Read the model definition and answer for the solid it produces. Units are mm, in the model's axes. A direction names the side the tool comes from. Coordinates: 2 decimals unless noted, no trailing zeros. Write each loop counter-clockwise with the first axis right and the second up, starting at its lowest first coordinate (ties: lowest second). Pieces come first, ordered by that corner, then holes.
1) Determine the mould class of faces 1 (the face through (131.79, 7.81, -1.73)), 2 (the face through (0, 17, -17)), 3 (the face through (96, 0, -11)) for opening direction X: +X half, -X half, draft (parallel to the pull), parting line (faces both ways), or undercut.
2) Each of these flat-tipped pins is pushed along its axis until it touches: pin 1 Ø10 at (x, z) = (55.5, 20.5) entering from -Y; pin 2 Ø16 at (x, y) = (91, -7) entering from +Z; pin 3 Ø4 at (x, z) = (100, 21) entering from +Y. Where does it stop, or does it pass through?
3) Which of the six approach directions +Z, -Z, +X, -X, +Y, -Y give full straight-line access (tool end or side, diameter ignored) to faces 4 (the face through (110, 16, 12)), 5 (the face through (110, -16, 12)), 6 (the face through (89.649, 0.528, 23.994))?
4) The part is cut by section A-A (x = 111.5). Determine the outline of the cut face in (y, z), then the cut area to 3 significant figures.
5) Find the intervals of material crossed by line 1 (Y direction, x = 133.25, z = 0); line 2 (Z direction, x = 45, y = 16); line 3 (Y direction, x = 56.75, z = 0), in increasing order.
6) The part is cut by section D-D (x = 26). Determine the outline of the cut face in (y, z).
7) The part is cut by section C-C (z = -5.5). Give the number of separate pieces and of enclosed holes in the cut face, then the cut area to 3 significant figures.
8) The part is cut by section B-B (y = 0). Determine the outline of the cut face in (x, z).
from build123d import *

# Parameters (mm, degrees)
CUT_EXTRUDE1_DEPTH = 151.996688705
SKETCH4_W          = 57
SKETCH4_H          = 22
CUT_EXTRUDE2_DEPTH = 156.357021604


with BuildPart() as part:
    # Sketch1 → Revolve1 (revolve)
    with BuildSketch(Plane(origin=(0, 0, 0), x_dir=(1, 0, 0), z_dir=(0, 1, 0)), mode=Mode.PRIVATE) as revolve1_sk:
        with BuildLine():
            Line((0, 0), (0, 40))
            Line((0, 40), (45, 24))
            Line((45, 24), (133.065732621, 24))
            ThreePointArc((133.065732621, 24), (138.23168958, 12.490837283), (140, 0))
            Line((140, 0), (0, 0))
        make_face()
    revolve(revolve1_sk.sketch.rotate(Axis((0, 0, 0), (1, 0, 0)), 180), axis=Axis((0, 0, 0), (1, 0, 0)))

    # Sketch2 → Cut-Extrude1 (cut, symmetric)
    with BuildSketch(Plane.XY):
        Polygon((469.549791622, 16), (137.05948169, 16), (67.5, 16), (0, 40), (-313.277254393, 151.387468229), (-199.953261752, 806.640776108), (582.873784263, 671.253307879), align=None)
    cut_extrude1 = extrude(amount=CUT_EXTRUDE1_DEPTH, both=True, mode=Mode.SUBTRACT)

    # Mirror1: Cut-Extrude1 across plane
    add(cut_extrude1.mirror(Plane.ZX), mode=Mode.SUBTRACT)

    # Sketch3 → Cut-Revolve2 (revolve, cut)
    with BuildSketch(Plane(origin=(0, 0, 0), x_dir=(1, 0, 0), z_dir=(0, 1, 0)), mode=Mode.PRIVATE) as cut_revolve2_sk:
        Polygon((0, 23.01873218), (0, 0), (140, 0), (140, 8), (42.240184255, 8), align=None)
    revolve(cut_revolve2_sk.sketch.rotate(Axis((0, 0, 0), (1, 0, 0)), 180), axis=Axis((0, 0, 0), (1, 0, 0)), mode=Mode.SUBTRACT)

    # Sketch4 → Cut-Extrude2 (cut, through all)
    with BuildSketch(Plane(origin=(0, 16, 0), x_dir=(1, 0, 0), z_dir=(0, 1, 0))):
        with Locations((96, 0)):
            Rectangle(SKETCH4_W, SKETCH4_H)
    extrude(amount=-CUT_EXTRUDE2_DEPTH, mode=Mode.SUBTRACT)


solid = part.part
Reported:
1. face 1: draft
1. face 2: -X half
1. face 3: undercut
2. pin 1: stops at y = -18.32
2. pin 2: stops at z = 24
2. pin 3: stops at y = 14.66
3. face 4: +Z, -Z, +X, +Y
3. face 5: +Z, -Z, +X, -Y
3. face 6: +Z, +X
4. outline: (-16, -17.89) arc R24 ccw to (16, -17.89) - (16, -11) - (-16, -11) - close; (-16, 11) - (16, 11) - (16, 17.89) arc R24 ccw to (-16, 17.89) - close
4. area: 709 mm2
5. line 1: y = -16 to -8, 8 to 16
5. line 2: z = -17.89 to 17.89
5. line 3: y = -19.82 to -8, 8 to 19.82
6. outline: circle Ø61.51 at (0, 0); hole circle Ø27.55 at (0, 0)
7. separate pieces: 4
7. enclosed holes: 0
7. area: 2,510 mm2
8. outline: (0, -40) - (45, -24) - (133.07, -24) arc R45 ccw to (139.28, -8) - (124.5, -8) - (124.5, -11) - (67.5, -11) - (67.5, -8) - (42.24, -8) - (0, -23.02) - close; (0, 23.02) - (42.24, 8) - (67.5, 8) - (67.5, 11) - (124.5, 11) - (124.5, 8) - (139.28, 8) arc R45 ccw to (133.07, 24) - (45, 24) - (0, 40) - close
